Build history of the part. All positions in model axes, mm. A direction names the side the tool comes from. Round coordinates to 2 decimals unless told otherwise and drop trailing zeros. Write each loop counter-clockwise with the first axis right and the second up, starting at its lowest first coordinate (ties: lowest second). Pieces come first, ordered by that corner, then holes. Notation, with made-up numbers: (6, 65) - (44, 65) arc R31 cw to (44, 90) - close; hole circle Ø5 at (-30.75, -14). An arc over 180 degrees is marked (long way). Write each question's results on one line, items separated by ' | '.
from build123d import *

# Parameters (mm, degrees)
SKETCH1_R           = 30
SKETCH1_R_2         = 2.5
BOSS_EXTRUDE1_DEPTH = 2
SKETCH2_R           = 10
SKETCH2_R_2         = 4
BOSS_EXTRUDE2_DEPTH = 15


with BuildPart() as part:
    # Sketch1 → Boss-Extrude1 (new body)
    with BuildSketch(Plane.XY):
        Circle(SKETCH1_R)
        with Locations((0, 23.75)):
            Circle(SKETCH1_R_2, mode=Mode.SUBTRACT)
        with Locations((20.56810334, 11.875)):
            Circle(SKETCH1_R_2, mode=Mode.SUBTRACT)
        with Locations((20.56810334, -11.875)):
            Circle(SKETCH1_R_2, mode=Mode.SUBTRACT)
        with Locations((0, -23.75)):
            Circle(SKETCH1_R_2, mode=Mode.SUBTRACT)
        with Locations((-20.56810334, -11.875)):
            Circle(SKETCH1_R_2, mode=Mode.SUBTRACT)
        with Locations((-20.56810334, 11.875)):
            Circle(SKETCH1_R_2, mode=Mode.SUBTRACT)
    extrude(amount=BOSS_EXTRUDE1_DEPTH)

    # Sketch2 → Boss-Extrude2 (add)
    with BuildSketch(Plane.XY.offset(2)):
        Circle(SKETCH2_R)
        Circle(SKETCH2_R_2, mode=Mode.SUBTRACT)
    extrude(amount=BOSS_EXTRUDE2_DEPTH)


solid = part.part
(1) Two-plate mould, pull along X, no slides. Class faces 1 (the cylindrical face through (-0.33, 26.23, 0.99)), 2 (the cylindrical face through (-2.17, -9.76, 9.4)), 3 (the flat face through (-0.1, -4.3, 17)): released by +X, released by -X, zero draft, split by the parting line, or undercut.
Worked answers:
face 1: undercut | face 2: split by the parting line | face 3: zero draft
(2) Slice it at D-D, the plane y = -23.75. Write the cut outline in (x, z).
Worked answers:
outline: (-18.33, 0) - (-2.5, 0) - (-2.5, 2) - (-18.33, 2) - close; (2.5, 0) - (18.33, 0) - (18.33, 2) - (2.5, 2) - close
(3) Slice it at A-A, the plane x = 0. Write the cut outline in (y, z), and give its area (3 significant figures).
Worked answers:
outline: (-30, 0) - (-26.25, 0) - (-26.25, 2) - (-30, 2) - close; (-21.25, 0) - (21.25, 0) - (21.25, 2) - (10, 2) - (10, 17) - (4, 17) - (4, 2) - (-4, 2) - (-4, 17) - (-10, 17) - (-10, 2) - (-21.25, 2) - close; (26.25, 0) - (30, 0) - (30, 2) - (26.25, 2) - close | area: 280 mm2
(4) Tool access for faces 4 (the flat face through (0, 0, 2)), 5 (the cylindrical face through (21.722, -14.093, 0.986)): list every direction of +Z, -Z, +X, -X, +Y, -Y with a clear straight run to the whole face (end or side of a thin tool).
Worked answers:
face 4: +Z | face 5: +Z, -Z
(5) Slice it at B-B, the plane y = 0. Write the cut outline in (x, z).
Worked answers:
outline: (-30, 0) - (30, 0) - (30, 2) - (10, 2) - (10, 17) - (4, 17) - (4, 2) - (-4, 2) - (-4, 17) - (-10, 17) - (-10, 2) - (-30, 2) - close
(6) Slice it at C-C, the plane z = 3. Write the cut outline in (x, y), and give its area (3 significant figures).
Worked answers:
outline: circle Ø20 at (0, 0); hole circle Ø8 at (0, 0) | area: 264 mm2
(7) Drill centre lines: probe 1 along Y at (x, z) = (0, 0.8); probe 2 along Z at (x, y) = (19, 3); probe 3 along Y at (x, z) = (5.5, 11.75). Where is each one in solid material? Low to high. Write a range as [from, to].
Worked answers:
probe 1: y = [-30, -26.25], [-21.25, 21.25], [26.25, 30] | probe 2: z = [0, 2] | probe 3: y = [-8.35, 8.35]
(8) Flat gauge pins, fed straight in: pin 1 Ø8 at (x, y) = (-14, 10.5) entering from +Z; pin 2 Ø4 at (x, y) = (0, 23.75) entering from +Z; pin 3 Ø4 at (y, z) = (-5, 4.5) entering from +X; pin 4 Ø10 at (y, z) = (23.5, 2) entering from +X. Where does each tip first touch, or does it go through?
Worked answers:
pin 1: stops at z = 2 | pin 2: passes through | pin 3: stops at x = 9.54 | pin 4: stops at x = 23.62
